CAD build for the part. Positions are in the model's coordinates, mm. Coordinates: 2 decimals unless noted, no trailing zeros. Loops run counter-clockwise (first coordinate to the right, second up) from the corner with the lowest first, then second, coordinate; pieces in that order, holes last. Notation, with made-up numbers: (6.25, 67.25) -> (58.25, 67.25) arc R12 cw to (58.25, 88.25) -> close; hole circle Ø7 at (40, -0.75). An arc over 180 degrees is marked (long way). Write each question's results on one line, items separated by ' | '.
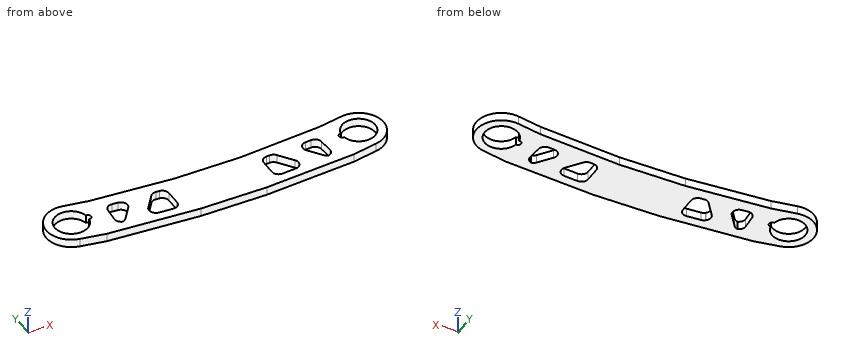
from build123d import *

# Parameters (mm, degrees)
Y_KSEKLIK_EKSTR_ZYON3_DEPTH = 5
KES_EKSTR_ZYON3_DEPTH       = 16
RADYUS1_R                   = 4
RADYUS1_OF_AYNALAMA1_R      = 4


with BuildPart() as part:
    # Çizim1 → Yükseklik-Ekstrüzyon3 (new body)
    with BuildSketch(Plane.XY):
        with BuildLine():
            Line((0, 14.764846508), (20, 14.764846508))
            Line((20, 14.764846508), (69.730204906, 18.686854932))
            Line((69.730204906, 18.686854932), (84.409297917, 21.275175082))
            ThreePointArc((84.409297917, 21.275175082), (101.971159912, 8.937394133), (89.578700393, -8.585926971))
            Line((89.578700393, -8.585926971), (74.828761414, -11.313435014))
            Line((74.828761414, -11.313435014), (20, -15.235443437))
            Line((20, -15.235443437), (0, -15.235443437))
            Line((0, -15.235443437), (0, 0))
            Line((0, 0), (0, 14.764846508))
        make_face()
    y_kseklik_ekstr_zyon3 = extrude(amount=Y_KSEKLIK_EKSTR_ZYON3_DEPTH)

    # Çizim2 → Kes-Ekstrüzyon3 (cut)
    with BuildSketch(Plane.XY):
        Polygon((28.695940883, -8.752311503), (42.731699056, -7.748306299), (46.735341753, -4.32569838), (36.65049886, 9.180616861), (28.695940883, 8.553274918), align=None)
        Polygon((49.583112015, 9.598582086), (61.257040732, -6.035946189), (65.565337221, -5.727765324), (64.37597588, 10.765231948), align=None)
        with BuildLine():
            ThreePointArc((77.201041987, 4.464811576), (97.059503272, 6.35268034), (77.201041987, 8.240549104))
            ThreePointArc((77.201041987, 8.240549104), (75.125188984, 6.35268034), (77.201041987, 4.464811576))
        make_face()
    kes_ekstr_zyon3 = extrude(amount=KES_EKSTR_ZYON3_DEPTH, mode=Mode.SUBTRACT)

    # Radyus1
    # the kernel refuses this fillet: 4 mm, written as the material it adds along each edge
    with BuildSketch(Plane(origin=(28.695940883, -8.752311503, 0), x_dir=(0, 1, 0), z_dir=(0, 0, 1))) as radyus1_piece_1:
        with BuildLine():
            CenterArc((RADYUS1_R * 1.07408709953, -RADYUS1_R), RADYUS1_R, 90, 94.091510037)
            Line((RADYUS1_R * 0.0766357332147, -RADYUS1_R * 1.07134964497), (0, 0))
            Line((0, 0), (RADYUS1_R * 1.07408709953, 0))
        make_face()
    extrude(amount=5)
    with BuildSketch(Plane(origin=(64.37597588, 10.765231948, 0), x_dir=(-0.9969045315308735, -0.0786215938099059, 0), z_dir=(0, 0, 1))) as radyus1_piece_2:
        with BuildLine():
            CenterArc((RADYUS1_R * 1.0067369642, RADYUS1_R), RADYUS1_R, 179.615297698, 90.384702302)
            Line((RADYUS1_R * 0.00675950517271, RADYUS1_R * 1.00671427137), (0, 0))
            Line((0, 0), (RADYUS1_R * 1.0067369642, 0))
        make_face()
    extrude(amount=5)
    with BuildSketch(Plane(origin=(49.583112015, 9.598582086, 0), x_dir=(0.9969045315308733, 0.07862159380990602, 0), z_dir=(0, 0, 1))) as radyus1_piece_3:
        with BuildLine():
            CenterArc((RADYUS1_R * 1.81293545135, -RADYUS1_R), RADYUS1_R, 90, 122.238478949)
            Line((RADYUS1_R * 0.967100347397, -RADYUS1_R * 1.53344444595), (0, 0))
            Line((0, 0), (RADYUS1_R * 1.81293545135, 0))
        make_face()
    extrude(amount=5)
    with BuildSketch(Plane(origin=(65.565337221, -5.727765324, 0), x_dir=(-0.07192633405101899, 0.9974099470478431, 0), z_dir=(0, 0, 1))) as radyus1_piece_4:
        with BuildLine():
            CenterArc((RADYUS1_R * 1.0005783418, RADYUS1_R), RADYUS1_R, 179.966873036, 90.033126964)
            Line((RADYUS1_R * 0.000578508947597, RADYUS1_R * 1.00057817457), (0, 0))
            Line((0, 0), (RADYUS1_R * 1.0005783418, 0))
        make_face()
    extrude(amount=5)
    with BuildSketch(Plane(origin=(46.735341753, -4.32569838, 0), x_dir=(-0.5982940894650627, 0.8012765955094231, 0), z_dir=(0, 0, 1))) as radyus1_piece_5:
        with BuildLine():
            CenterArc((RADYUS1_R * 0.936136482984, RADYUS1_R), RADYUS1_R, 183.778435906, 86.221564094)
            Line((-RADYUS1_R * 0.0616898577771, RADYUS1_R * 0.934101641269), (0, 0))
            Line((0, 0), (RADYUS1_R * 0.936136482984, 0))
        make_face()
    extrude(amount=5)
    with BuildSketch(Plane(origin=(36.65049886, 9.180616861, 0), x_dir=(-0.9969045315308735, -0.07862159380990552, 0), z_dir=(0, 0, 1))) as radyus1_piece_6:
        with BuildLine():
            CenterArc((RADYUS1_R * 0.551591618585, RADYUS1_R), RADYUS1_R, 212.238478949, 57.761521051)
            Line((-RADYUS1_R * 0.294243485369, RADYUS1_R * 0.466555554046), (0, 0))
            Line((0, 0), (RADYUS1_R * 0.551591618585, 0))
        make_face()
    extrude(amount=5)
    with BuildSketch(Plane(origin=(28.695940883, 8.553274918, 0), x_dir=(0, -1, 0), z_dir=(0, 0, 1))) as radyus1_piece_7:
        with BuildLine():
            CenterArc((RADYUS1_R * 0.924239359987, RADYUS1_R), RADYUS1_R, 184.509339304, 85.490660696)
            Line((-RADYUS1_R * 0.072665171544, RADYUS1_R * 0.92137840619), (0, 0))
            Line((0, 0), (RADYUS1_R * 0.924239359987, 0))
        make_face()
    extrude(amount=5)
    with BuildSketch(Plane(origin=(42.731699056, -7.748306299, 0), x_dir=(0.7601082947002393, 0.6497964145237292, 0), z_dir=(0, 0, 1))) as radyus1_piece_8:
        with BuildLine():
            CenterArc((RADYUS1_R * 0.32911927964, RADYUS1_R), RADYUS1_R, 233.565255877, 36.434744123)
            Line((-RADYUS1_R * 0.26478758489, RADYUS1_R * 0.195466199427), (0, 0))
            Line((0, 0), (RADYUS1_R * 0.32911927964, 0))
        make_face()
    extrude(amount=5)
    with BuildSketch(Plane(origin=(61.257040732, -6.035946189, 0), x_dir=(0.9974513663147319, 0.07134964496670383, 0), z_dir=(0, 0, 1))) as radyus1_piece_9:
        with BuildLine():
            CenterArc((RADYUS1_R * 0.546845511805, RADYUS1_R), RADYUS1_R, 212.656308216, 57.343691784)
            Line((-RADYUS1_R * 0.295076994051, RADYUS1_R * 0.460401543615), (0, 0))
            Line((0, 0), (RADYUS1_R * 0.546845511805, 0))
        make_face()
    extrude(amount=5)

    # Aynalama1: Yükseklik-Ekstrüzyon3, Kes-Ekstrüzyon3 across plane
    add(y_kseklik_ekstr_zyon3.mirror(Plane(origin=(0, 0, 5), x_dir=(0, 0, 1), z_dir=(1, 0, 0))))
    add(kes_ekstr_zyon3.mirror(Plane(origin=(0, 0, 5), x_dir=(0, 0, 1), z_dir=(1, 0, 0))), mode=Mode.SUBTRACT)

    # Radyus1 of Aynalama1
    # the kernel refuses this fillet: 4 mm, written as the material it adds along each edge
    with BuildSketch(Plane(origin=(-28.695940883, -8.752311503, 0), x_dir=(-0.9974513663147319, 0.07134964496670435, 0), z_dir=(0, 0, 1))) as radyus1_of_aynalama1_piece_1:
        with BuildLine():
            CenterArc((RADYUS1_OF_AYNALAMA1_R * 1.07408709953, -RADYUS1_OF_AYNALAMA1_R), RADYUS1_OF_AYNALAMA1_R, 90, 94.091510037)
            Line((RADYUS1_OF_AYNALAMA1_R * 0.0766357332147, -RADYUS1_OF_AYNALAMA1_R * 1.07134964497), (0, 0))
            Line((0, 0), (RADYUS1_OF_AYNALAMA1_R * 1.07408709953, 0))
        make_face()
    extrude(amount=5)
    with BuildSketch(Plane(origin=(-64.37597588, 10.765231948, 0), x_dir=(-0.07192633405101888, -0.9974099470478431, 0), z_dir=(0, 0, 1))) as radyus1_of_aynalama1_piece_2:
        with BuildLine():
            CenterArc((RADYUS1_OF_AYNALAMA1_R * 1.0067369642, RADYUS1_OF_AYNALAMA1_R), RADYUS1_OF_AYNALAMA1_R, 179.615297698, 90.384702302)
            Line((RADYUS1_OF_AYNALAMA1_R * 0.00675950517271, RADYUS1_OF_AYNALAMA1_R * 1.00671427137), (0, 0))
            Line((0, 0), (RADYUS1_OF_AYNALAMA1_R * 1.0067369642, 0))
        make_face()
    extrude(amount=5)
    with BuildSketch(Plane(origin=(-49.583112015, 9.598582086, 0), x_dir=(-0.5982940894650629, -0.801276595509423, 0), z_dir=(0, 0, 1))) as radyus1_of_aynalama1_piece_3:
        with BuildLine():
            CenterArc((RADYUS1_OF_AYNALAMA1_R * 1.81293545135, -RADYUS1_OF_AYNALAMA1_R), RADYUS1_OF_AYNALAMA1_R, 90, 122.238478949)
            Line((RADYUS1_OF_AYNALAMA1_R * 0.967100347397, -RADYUS1_OF_AYNALAMA1_R * 1.53344444595), (0, 0))
            Line((0, 0), (RADYUS1_OF_AYNALAMA1_R * 1.81293545135, 0))
        make_face()
    extrude(amount=5)
    with BuildSketch(Plane(origin=(-65.565337221, -5.727765324, 0), x_dir=(0.9974513663147317, -0.07134964496670429, 0), z_dir=(0, 0, 1))) as radyus1_of_aynalama1_piece_4:
        with BuildLine():
            CenterArc((RADYUS1_OF_AYNALAMA1_R * 1.0005783418, RADYUS1_OF_AYNALAMA1_R), RADYUS1_OF_AYNALAMA1_R, 179.966873036, 90.033126964)
            Line((RADYUS1_OF_AYNALAMA1_R * 0.000578508947597, RADYUS1_OF_AYNALAMA1_R * 1.00057817457), (0, 0))
            Line((0, 0), (RADYUS1_OF_AYNALAMA1_R * 1.0005783418, 0))
        make_face()
    extrude(amount=5)
    with BuildSketch(Plane(origin=(-46.735341753, -4.32569838, 0), x_dir=(0.7601082947002414, -0.6497964145237266, 0), z_dir=(0, 0, 1))) as radyus1_of_aynalama1_piece_5:
        with BuildLine():
            CenterArc((RADYUS1_OF_AYNALAMA1_R * 0.936136482984, RADYUS1_OF_AYNALAMA1_R), RADYUS1_OF_AYNALAMA1_R, 183.778435906, 86.221564094)
            Line((-RADYUS1_OF_AYNALAMA1_R * 0.0616898577771, RADYUS1_OF_AYNALAMA1_R * 0.934101641269), (0, 0))
            Line((0, 0), (RADYUS1_OF_AYNALAMA1_R * 0.936136482984, 0))
        make_face()
    extrude(amount=5)
    with BuildSketch(Plane(origin=(-36.65049886, 9.180616861, 0), x_dir=(-0.5982940894650631, -0.8012765955094229, 0), z_dir=(0, 0, 1))) as radyus1_of_aynalama1_piece_6:
        with BuildLine():
            CenterArc((RADYUS1_OF_AYNALAMA1_R * 0.551591618585, RADYUS1_OF_AYNALAMA1_R), RADYUS1_OF_AYNALAMA1_R, 212.238478949, 57.761521051)
            Line((-RADYUS1_OF_AYNALAMA1_R * 0.294243485369, RADYUS1_OF_AYNALAMA1_R * 0.466555554046), (0, 0))
            Line((0, 0), (RADYUS1_OF_AYNALAMA1_R * 0.551591618585, 0))
        make_face()
    extrude(amount=5)
    with BuildSketch(Plane(origin=(-28.695940883, 8.553274918, 0), x_dir=(-0.9969045315308733, 0.07862159380990529, 0), z_dir=(0, 0, 1))) as radyus1_of_aynalama1_piece_7:
        with BuildLine():
            CenterArc((RADYUS1_OF_AYNALAMA1_R * 0.924239359987, RADYUS1_OF_AYNALAMA1_R), RADYUS1_OF_AYNALAMA1_R, 184.509339304, 85.490660696)
            Line((-RADYUS1_OF_AYNALAMA1_R * 0.072665171544, RADYUS1_OF_AYNALAMA1_R * 0.92137840619), (0, 0))
            Line((0, 0), (RADYUS1_OF_AYNALAMA1_R * 0.924239359987, 0))
        make_face()
    extrude(amount=5)
    with BuildSketch(Plane(origin=(-42.731699056, -7.748306299, 0), x_dir=(0.9974513663147319, -0.07134964496670414, 0), z_dir=(0, 0, 1))) as radyus1_of_aynalama1_piece_8:
        with BuildLine():
            CenterArc((RADYUS1_OF_AYNALAMA1_R * 0.32911927964, RADYUS1_OF_AYNALAMA1_R), RADYUS1_OF_AYNALAMA1_R, 233.565255877, 36.434744123)
            Line((-RADYUS1_OF_AYNALAMA1_R * 0.26478758489, RADYUS1_OF_AYNALAMA1_R * 0.195466199427), (0, 0))
            Line((0, 0), (RADYUS1_OF_AYNALAMA1_R * 0.32911927964, 0))
        make_face()
    extrude(amount=5)
    with BuildSketch(Plane(origin=(-61.257040732, -6.035946189, 0), x_dir=(0.5982940894650642, 0.8012765955094219, 0), z_dir=(0, 0, 1))) as radyus1_of_aynalama1_piece_9:
        with BuildLine():
            CenterArc((RADYUS1_OF_AYNALAMA1_R * 0.546845511805, RADYUS1_OF_AYNALAMA1_R), RADYUS1_OF_AYNALAMA1_R, 212.656308216, 57.343691784)
            Line((-RADYUS1_OF_AYNALAMA1_R * 0.295076994051, RADYUS1_OF_AYNALAMA1_R * 0.460401543615), (0, 0))
            Line((0, 0), (RADYUS1_OF_AYNALAMA1_R * 0.546845511805, 0))
        make_face()
    extrude(amount=5)


solid = part.part
1) Slice it at C-C (x = 3). Write the cut outline in (y, z), then the cut area to 3 significant figures.
Outcome:
outline: (-15.24, 0) -> (14.76, 0) -> (14.76, 5) -> (-15.24, 5) -> close | area: 150 mm^2
2) Drill centre lines: L1, parallel to X at y = 12, z = 2.2; L2, parallel to X at y = -7, z = 3.6; L3, parallel to Y at x = -3, z = 3.05. Where is each one in solid material? Low to high. Write a range as from..to.
Outcome:
L1: x = -101.1..-95.32, -78.76..78.76, 95.32..101.1 | L2: x = -94.2..-43.6, -29.61..29.61, 43.6..94.2 | L3: y = -15.24..14.76
3) Pin check, flat tips, straight feed: pin 1 (1.5 mm diameter, centred on x = 53.5, z = 1.5, fed in from +Y); pin 2 (1.5 mm diameter, centred on y = 1, z = 3, fed in from -X); pin 3 (1 mm diameter, centred on y = -8, z = 0.5, fed in from -X); pin 4 (4.5 mm diameter, centred on x = 77.02, y = 6.35, fed in from +Z). Stop position of each tip, or through.
Outcome:
pin 1: stops at y = 17.47 | pin 2: stops at x = -101.48 | pin 3: stops at x = -93.18 | pin 4: stops at z = 5
4) Slice it at D-D (z = 3.15). Count the separate pieces of the cut face and the enclosed holes in it, then the cut area to 3 significant figures.
Outcome:
separate pieces: 1 | enclosed holes: 6 | area: 4,620 mm^2
5) Slice it at A-A (y = 12.5). Write the cut outline in (x, z).
Outcome:
outline: (-100.89, 0) -> (-94.95, 0) -> (-94.95, 5) -> (-100.89, 5) -> close; (-79.13, 0) -> (79.13, 0) -> (79.13, 5) -> (-79.13, 5) -> close; (94.95, 0) -> (100.89, 0) -> (100.89, 5) -> (94.95, 5) -> close
6) Slice it at B-B (y = 0.5). Write the cut outline in (x, z), then the cut area to 3 significant figures.
Outcome:
outline: (-101.02, 0) -> (-95.17, 0) -> (-95.17, 5) -> (-101.02, 5) -> close; (-78.91, 0) -> (-65.12, 0) -> (-65.12, 5) -> (-78.91, 5) -> close; (-56.38, 0) -> (-43.13, 0) -> (-43.13, 5) -> (-56.38, 5) -> close; (-28.7, 0) -> (28.7, 0) -> (28.7, 5) -> (-28.7, 5) -> close; (43.13, 0) -> (56.38, 0) -> (56.38, 5) -> (43.13, 5) -> close; (65.12, 0) -> (78.91, 0) -> (78.91, 5) -> (65.12, 5) -> close; (95.17, 0) -> (101.02, 0) -> (101.02, 5) -> (95.17, 5) -> close | area: 616 mm^2
